Autodesk Inventor part; units mm, degrees
ref_plane "YZ Plane" through (0, 0, 0) normal (1, 0, 0) x (0, 1, 0)
ref_plane "XZ Plane" through (0, 0, 0) normal (0, 1, 0) x (-1, 0, 0)
ref_plane "XY Plane" through (0, 0, 0) normal (0, 0, 1) x (1, 0, 0)
sketch "Sketch3" plane through (0, 0, 0) normal (0, 0, 1) x (1, 0, 0)
  line L0 (3, 4) -> (128, 4)
  line L1 (128, 4) -> (128, 59)
  line L2 (128, 59) -> (3, 59)
  line L3 (3, 59) -> (3, 4)
  point P0 (0, 0)
  dimension "d0" = 125
  dimension "d1" = 55
extrude "Extrusion1" add sketch "Sketch3" along normal blind 5
sketch "Sketch7" plane through (0, 0, 5) normal (0, 0, 1) x (1, 0, 0)
  line L0 (128, 4) -> (128, 59)
  line L1 (0, 4) -> (128, 4)
  line L2 (128, 59) -> (53, 59)
  line L3 (53, 59) -> (53, 4)
  line L4 (53, 4) -> (128, 4)
  line L5 (128, 4) -> (128, 59)
  point P0 (0, 0)
  dimension "d20" = 75
extrude "Extrusion3" add sketch "Sketch7" along normal blind 10
sketch "Sketch8" plane through (0, 0, 15) normal (0, 0, 1) x (1, 0, 0)
  line L0 (53, 59) -> (53, 4)
  line L1 (53, 4) -> (53, 13)
  line L2 (53, 13) -> (118, 13)
  line L3 (118, 13) -> (118, 40)
  line L4 (118, 40) -> (53, 40)
  line L5 (53, 40) -> (53, 13)
  point P0 (0, 0)
  dimension "d23" = 9
  dimension "d24" = 65
  dimension "d25" = 27
extrude "Extrusion4" cut sketch "Sketch8" against normal blind 10
sketch "Sketch9" plane through (0, 0, 15) normal (0, 0, 1) x (1, 0, 0)
  line L0 (53, 40) -> (118, 40)
  line L1 (118, 13) -> (53, 13)
  line L2 (118, 40) -> (103, 40)
  line L3 (103, 40) -> (103, 13)
  line L4 (103, 13) -> (118, 13)
  line L5 (118, 13) -> (118, 40)
  point P0 (0, 0)
  dimension "d28" = 15
extrude "Extrusion5" cut sketch "Sketch9" against normal blind 20
sketch "Sketch12" plane through (0, 0, 5) normal (0, 0, 1) x (1, 0, 0)
  line L0 (0, 0) -> (0, 63)
  line L1 (0, 63) -> (128, 63)
  line L2 (128, 63) -> (128, 59)
  line L3 (3, 59) -> (128, 59)
  line L4 (128, 59) -> (3, 59)
  line L5 (3, 4) -> (3, 59)
  line L6 (3, 59) -> (3, 4)
  line L7 (128, 59) -> (128, 4)
  line L8 (3, 4) -> (128, 4)
  line L9 (128, 4) -> (128, 0)
  line L10 (128, 0) -> (0, 0)
  dimension "d35" = 63
  dimension "d36" = 128
  dimension "d37" = 90
extrude "Extrusion6" add sketch "Sketch12" along normal blind 10 and the other way blind 5 contours L0 L1 L2 L3 L5 L8 L9 L10
sketch "Sketch14" plane through (0, 0, 5) normal (0, 0, 1) x (1, 0, 0)
  line L0 (53, 40) -> (103, 40)
  line L1 (53, 40) -> (55, 40)
  line L2 (55, 40) -> (55, 59)
  line L3 (55, 59) -> (53, 59)
  line L4 (53, 59) -> (53, 40)
  point P0 (0, 0)
  dimension "d42" = 2
extrude "Extrusion7" cut sketch "Sketch14" along normal blind 10
sketch "Sketch15" plane through (0, 0, 15) normal (0, 0, 1) x (1, 0, 0)
  line L0 (53, 4) -> (53, 13)
  line L1 (53, 13) -> (55, 13)
  line L2 (55, 13) -> (55, 4)
  line L3 (55, 4) -> (53, 4)
  line L4 (53, 4) -> (53, 13)
  point P0 (0, 0)
  dimension "d45" = 2
extrude "Extrusion8" cut sketch "Sketch15" against normal blind 10
sketch "Sketch17" plane through (0, 0, 15) normal (0, 0, 1) x (1, 0, 0)
  point P0 (0, 0)
properties part number "Case"
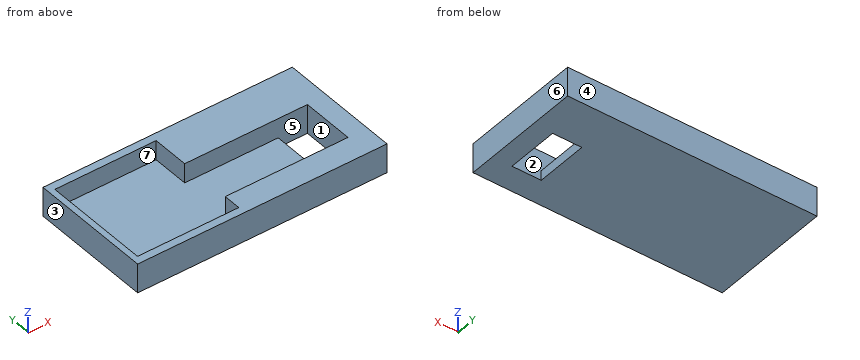
For this review, take the finished solid that the model builds, in its own axes (mm). Face numbers are marked on the shaded views. A direction names the side the tool comes from. Round coordinates to 2 decimals unless told otherwise and drop trailing zeros. Order: outer loops, then holes, each group sorted by start corner. A loop starts at its lowest first (then second) coordinate and runs counter-clockwise, first axis right, second up. Notation, with made-up numbers: (-29, -24.75) -> (8, -24.75) arc R15 cw to (8, -17.75) -> close; hole circle Ø8 at (-12.75, 27). An arc over 180 degrees is marked (long way). Use a Markdown table: item, result.
Item 1: For line 1 along X through (y, z) = (18, 1.5); line 2 along X through (y, z) = (12, 5.25); line 3 along Y through (x, z) = (113.5, 1.5), list the stretches that pass through material, from the lowest coordinate up. Write a range as [from, to].
Resolved:
| item | result |
|---|---|
| line 1 | x = [0, 103], [118, 128] |
| line 2 | x = [0, 3], [55, 128] |
| line 3 | y = [0, 13], [40, 63] |
Item 2: Take a section at C-C (x = 24.5). State the section outline as (y, z) points.
Resolved:
| item | result |
|---|---|
| outline | (0, 0) -> (63, 0) -> (63, 15) -> (59, 15) -> (59, 5) -> (4, 5) -> (4, 15) -> (0, 15) -> close |
Item 3: Machinability: for the marked faces 1, 2 and 3, which of the approach directions +Z, -Z, +X, -X, +Y, -Y give a long, thin tool a straight path to every point of the face, cutting with its end or side? Answer none if there is none.
Resolved:
| item | result |
|---|---|
| face 1 | +Z, -Z |
| face 2 | +Z |
| face 3 | +Z, -Z, -X, +Y, -Y |
Item 4: For pin 1 (1.5 mm diameter, centred on x = 70, y = 33, fed in from +Z), flat-tipped, find the tip position at first contact; note if it passes through.
Resolved:
| item | result |
|---|---|
| pin 1 | stops at z = 5 |
Item 5: Draft analysis for pull direction X (two halves, no side actions). For the marked faces 4, 5, 6 and 7, state which applies: +X half, -X half, draft (parallel to the pull), parting line (faces both ways), or undercut.
Resolved:
| item | result |
|---|---|
| face 4 | draft |
| face 5 | undercut |
| face 6 | +X half |
| face 7 | undercut |
Item 6: Take a section at D-D (y = 45.5). State the section outline as (x, z) points, plus the area to 3 significant figures.
Resolved:
| item | result |
|---|---|
| outline | (0, 0) -> (128, 0) -> (128, 15) -> (55, 15) -> (55, 5) -> (3, 5) -> (3, 15) -> (0, 15) -> close |
| area | 1,400 mm² |
Item 7: Take a section at A-A (z = 3). State the section outline as (x, y) points, plus the area to 3 significant figures.
Resolved:
| item | result |
|---|---|
| outline | (0, 0) -> (128, 0) -> (128, 63) -> (0, 63) -> close; hole (103, 13) -> (118, 13) -> (118, 40) -> (103, 40) -> close |
| area | 7,660 mm² |
Item 8: Take a section at B-B (x = 110.5). State the section outline as (y, z) points, plus the area to 3 significant figures.
Resolved:
| item | result |
|---|---|
| outline | (0, 0) -> (13, 0) -> (13, 15) -> (0, 15) -> close; (40, 0) -> (63, 0) -> (63, 15) -> (40, 15) -> close |
| area | 540 mm² |
